Could you check a few things on this drawing? It's one solid part, dimensions in mm from its lowest x, y, z. Coordinates: 2 decimals unless noted, no trailing zeros. Loops run counter-clockwise (first coordinate to the right, second up) from the corner with the lowest first, then second, coordinate; pieces in that order, holes last. Notation, with made-up numbers: M 85,44.25 L 106,44.25 A21 cw 106,72.25 Z; hole C 11.25,-24 d4. An arc over 180 degrees is marked long. Answer as a JSON object with one key per item and string values. Group by question number.
Item 1: Suppose I cut it at D-D (x = 37). Write out the boundary of the cut face in (y, z), then the cut area to 3 significant figures.
Item 2: We'd pull the mould along Y, two halves only. Please class the marked faces 1, 2 and 3: +Y half, -Y half, draft (parallel to the pull), parting line (faces both ways), or undercut.
Item 3: Suppose I cut it at A-A (x = 47.5). Write out the boundary of the cut face in (y, z), then the cut area to 3 significant figures.
Item 4: If I drill on line 1 (Y direction, x = 47.5, z = 2.85); line 2 (Y direction, x = 85, z = 2.95); line 3 (X direction, y = 17, z = 3.3), over which ranges is the centre line in solid material (lowest first)?
Item 5: Suppose I cut it at B-B (y = 19). Write out the boundary of the cut face in (x, z).
Item 6: Suppose I cut it at C-C (z = 1.5). Write out the boundary of the cut face in (x, y), then the cut area to 3 significant figures.
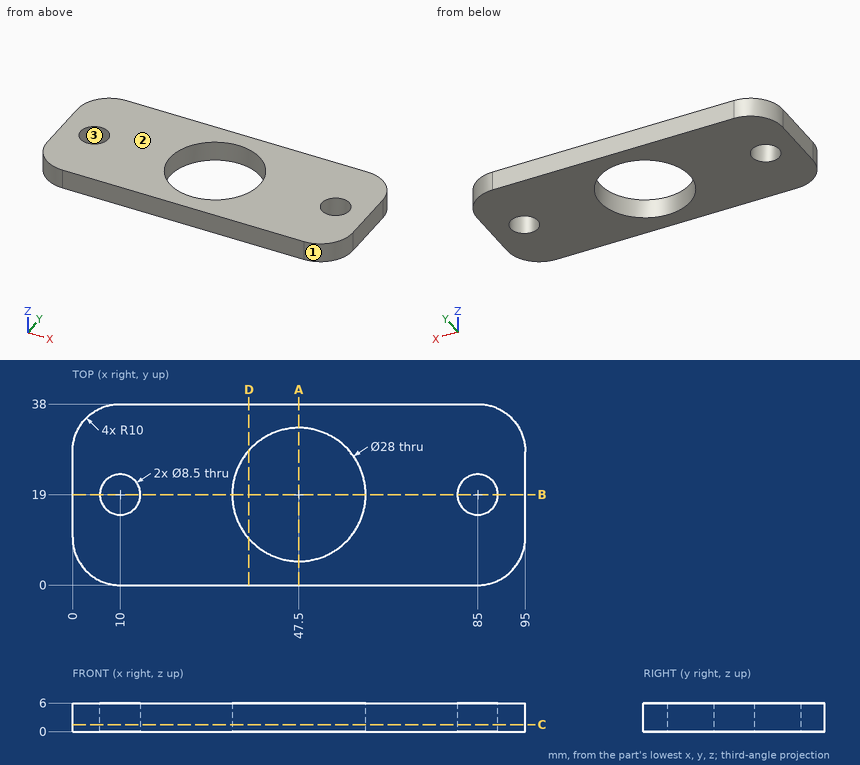
From the geometry:
{
 "1": {"outline": "M 0,0 L 9.74,0 L 9.74,6 L 0,6 Z; M 28.26,0 L 38,0 L 38,6 L 28.26,6 Z", "area": "117 mm2"},
 "2": {"face 1": "-Y half", "face 2": "draft", "face 3": "undercut"},
 "3": {"outline": "M 0,0 L 5,0 L 5,6 L 0,6 Z; M 33,0 L 38,0 L 38,6 L 33,6 Z", "area": "60.0 mm2"},
 "4": {"line 1": "0 to 5, 33 to 38", "line 2": "0 to 14.75, 23.25 to 38", "line 3": "0 to 6.25, 13.75 to 33.64, 61.36 to 81.25, 88.75 to 95"},
 "5": {"outline": "M 0,0 L 5.75,0 L 5.75,6 L 0,6 Z; M 14.25,0 L 33.5,0 L 33.5,6 L 14.25,6 Z; M 61.5,0 L 80.75,0 L 80.75,6 L 61.5,6 Z; M 89.25,0 L 95,0 L 95,6 L 89.25,6 Z"},
 "6": {"outline": "M 0,10 A10 ccw 10,0 L 85,0 A10 ccw 95,10 L 95,28 A10 ccw 85,38 L 10,38 A10 ccw 0,28 Z; hole C 10,19 d8.5; hole C 47.5,19 d28; hole C 85,19 d8.5", "area": "2,790 mm2"}
}
